The listing builds one solid part. Answer for the finished solid, in the listing's coordinates (mm). Face numbers are marked on the shaded views. A direction names the side the tool comes from. Coordinates: 2 decimals unless noted, no trailing zeros. Order: outer loops, then holes, each group sorted by start corner. A loop starts at its lowest first (then second) coordinate and runs counter-clockwise, first axis right, second up. Notation, with made-up numbers: (21, 37.5) -> (79, 37.5) arc R13 ccw to (79, 55.5) -> close; hole circle Ø7 at (-24.5, 50.5). An arc over 180 degrees is marked (long way). One line per question, with ' | ' between items.
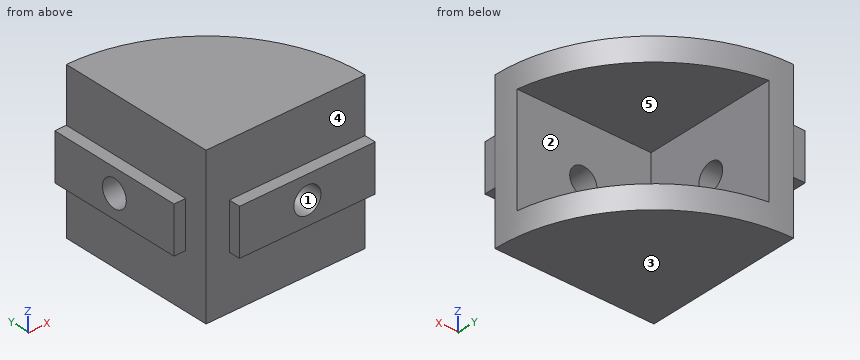
from build123d import *

# Parameters (mm, degrees)
Y_KSEKLIK_EKSTR_ZYON1_DEPTH = 20
KES_EKSTR_ZYON1_START       = 3
IZIM2_W                     = 14
IZIM2_H                     = 17.5
KES_EKSTR_ZYON1_DEPTH       = 33.220732531
IZIM6_W                     = 6
IZIM6_H                     = 1.5
Y_KSEKLIK_EKSTR_ZYON3_DEPTH = 17.5
SKETCH_2_R                  = 1.75
CUT_EXTRUDE_2_DEPTH         = 5
SKETCH_3_W                  = 6
SKETCH_3_H                  = 17.5
EXTRUDE_1_DEPTH             = 1.5
SKETCH_4_R                  = 1.75
CUT_EXTRUDE_3_DEPTH         = 5


with BuildPart() as part:
    # Çizim1 → Yükseklik-Ekstrüzyon1 (new body)
    with BuildSketch(Plane.XY):
        with BuildLine():
            Line((0, 20.5), (0, 0))
            Line((0, 0), (20.5, 0))
            ThreePointArc((20.5, 0), (14.495689014, 14.495689014), (0, 20.5))
        make_face()
    extrude(amount=Y_KSEKLIK_EKSTR_ZYON1_DEPTH)

    # Çizim2 → Kes-Ekstrüzyon1 (cut, through all)
    with BuildSketch(Plane(origin=(0, 0, 0), x_dir=(0, 0, -1), z_dir=(1, 0, 0)).offset(KES_EKSTR_ZYON1_START)):
        with Locations((-10, 11.75)):
            Rectangle(IZIM2_W, IZIM2_H)
    extrude(amount=KES_EKSTR_ZYON1_DEPTH, mode=Mode.SUBTRACT)

    # Çizim6 → Yükseklik-Ekstrüzyon3 (add, through all)
    with BuildSketch(Plane(origin=(3, 0, 0), x_dir=(0, 0, -1), z_dir=(1, 0, 0))):
        with Locations((-10, -0.75)):
            Rectangle(IZIM6_W, IZIM6_H)
    extrude(amount=Y_KSEKLIK_EKSTR_ZYON3_DEPTH)

    # Эскиз2 → Вырез-Вытянуть2 (cut)
    with BuildSketch(Plane.XZ.offset(1.5)):
        with Locations(Location((11.75, 10, 0), (0, 0, 270))):
            Circle(SKETCH_2_R)
    extrude(amount=-CUT_EXTRUDE_2_DEPTH, mode=Mode.SUBTRACT)

    # Эскиз3 → Бобышка-Вытянуть1 (add)
    with BuildSketch(Plane.ZY):
        with Locations((10, 11.75)):
            Rectangle(SKETCH_3_W, SKETCH_3_H)
    extrude(amount=EXTRUDE_1_DEPTH)

    # Эскиз4 → Вырез-Вытянуть3 (cut)
    with BuildSketch(Plane.ZY.offset(1.5)):
        with Locations(Location((10, 11.75, 0), (0, 0, 270))):
            Circle(SKETCH_4_R)
    extrude(amount=-CUT_EXTRUDE_3_DEPTH, mode=Mode.SUBTRACT)


solid = part.part
Item 1: Each of these flat-tipped pins is pushed along its axis until it touches: pin 1 Ø1.2 at (y, z) = (-1, 9.5) entering from -X; pin 2 Ø3 at (y, z) = (11.75, 10) entering from +X; pin 3 Ø0.8 at (x, y) = (12.5, -1) entering from +Z; pin 4 Ø4 at (y, z) = (8.5, 13) entering from +X. Where does it stop, or does it pass through?
Computed values:
pin 1: stops at x = 3 | pin 2: passes through | pin 3: stops at z = 13 | pin 4: stops at x = 3
Item 2: Section A-A, the plane z = 10 is taken. Give the vertices of the cut face in (x, y), plus the area to 3 significant figures.
Computed values:
outline: (-1.5, 3) -> (0, 3) -> (0, 0) -> (3, 0) -> (3, -1.5) -> (10, -1.5) -> (10, 3) -> (3, 3) -> (3, 10) -> (-1.5, 10) -> close; (-1.5, 13.5) -> (3, 13.5) -> (3, 20.28) arc R20.5 ccw to (0, 20.5) -> (-1.5, 20.5) -> close; (13.5, -1.5) -> (20.5, -1.5) -> (20.5, 0) arc R20.5 ccw to (20.28, 3) -> (13.5, 3) -> close | area: 135 mm^2
Item 3: Section D-D, the plane z = 7.75 is taken. Give the vertices of the cut face in (x, y), plus the area to 3 significant figures.
Computed values:
outline: (-1.5, 3) -> (0, 3) -> (0, 0) -> (3, 0) -> (3, -1.5) -> (20.5, -1.5) -> (20.5, 0) arc R20.5 ccw to (20.28, 3) -> (3, 3) -> (3, 20.28) arc R20.5 ccw to (0, 20.5) -> (-1.5, 20.5) -> close | area: 166 mm^2
Item 4: Determine the mould class of the marked faces 3, 4 and 5 for opening direction Z: pulls with the +Z half, pulls with the -Z half, needs draft (parallel to the pull), parting line crosses it, or undercut.
Computed values:
face 3: pulls with the -Z half | face 4: needs draft | face 5: undercut
Item 5: Section B-B, the plane y = 11.75 is taken. Give the vertices of the cut face in (x, z), plus the area to 3 significant figures.
Computed values:
outline: (-1.5, 7) -> (0, 7) -> (0, 0) -> (16.8, 0) -> (16.8, 3) -> (3, 3) -> (3, 8.25) -> (-1.5, 8.25) -> close; (-1.5, 11.75) -> (3, 11.75) -> (3, 17) -> (16.8, 17) -> (16.8, 20) -> (0, 20) -> (0, 13) -> (-1.5, 13) -> close | area: 136 mm^2
Item 6: For the marked faces 1 and 2, determine the directions among +Z, -Z, +X, -X, +Y, -Y from which every point of the face is accessible in a straight line to the end or side of a thin tool.
Computed values:
face 1: +Y, -Y | face 2: +X, +Y
Item 7: Find the intervals of material crossed by L1, parallel to Z at x = 1.6, y = 11.75; L2, parallel to Z at x = 12.5, y = 10; L3, parallel to Y at x = 13, z = 3.5, in increasing order.
Computed values:
L1: z = 0 to 8.25, 11.75 to 20 | L2: z = 0 to 3, 17 to 20 | L3: y = 0 to 3
